```python
from build123d import *

# Parameters (mm, degrees)
BOSS_EXTRUDE1_DEPTH          = 44
SKETCH3_W                    = 50
SKETCH3_H                    = 50
BOSS_EXTRUDE2_DEPTH          = 11
SKETCH4_R                    = 21.25
SKETCH4_R_2                  = 12.25
CUT_EXTRUDE1_DEPTH           = 4
SKETCH5_3_R                  = 1.6
CUT_EXTRUDE3_DEPTH           = 20
SKETCH5_R                    = 2.5
CUT_EXTRUDE4_DEPTH           = 5
FILLET2_R                    = 15
SKETCH8_R                    = 3
CUT_EXTRUDE5_DEPTH           = 15
SCHIZZO2_W                   = 250
SCHIZZO2_H                   = 250
SCHIZZO2_W_2                 = 25.273765435
SCHIZZO2_H_2                 = 26.723899517
ESTRUSIONE_ESTRUSIONE1_DEPTH = 9
SCHIZZO5_W                   = 250
SCHIZZO5_H                   = 250
SCHIZZO5_W_2                 = 121.71
SCHIZZO5_H_2                 = 121.711825152
ESTRUSIONE_ESTRUSIONE2_DEPTH = 50


with BuildPart() as part:
    # Sketch1 → Boss-Extrude1 (new body)
    with BuildSketch(Plane.XY):
        Polygon((-22.5, 0), (22.5, 0), (18, 9), (-18, 9), align=None)
    extrude(amount=BOSS_EXTRUDE1_DEPTH)

    # Sketch3 → Boss-Extrude2 (add)
    with BuildSketch(Plane(origin=(0, 9, 0), x_dir=(1, 0, 0), z_dir=(0, 1, 0))):
        with Locations((0, -22)):
            Rectangle(SKETCH3_W, SKETCH3_H)
    extrude(amount=BOSS_EXTRUDE2_DEPTH)

    # Sketch4 → Cut-Extrude1 (cut)
    with BuildSketch(Plane(origin=(0, 20, 0), x_dir=(1, 0, 0), z_dir=(0, 1, 0))):
        with Locations((0, -22)):
            Circle(SKETCH4_R)
        with Locations((0, -22)):
            Circle(SKETCH4_R_2, mode=Mode.SUBTRACT)
    extrude(amount=-CUT_EXTRUDE1_DEPTH, mode=Mode.SUBTRACT)

    # Sketch5<3> → Cut-Extrude3 (cut)
    with BuildSketch(Plane(origin=(0, 20, 0), x_dir=(1, 0, 0), z_dir=(0, 1, 0))):
        with Locations((0, -15)):
            Circle(SKETCH5_3_R)
        with Locations((-7, -22)):
            Circle(SKETCH5_3_R)
        with Locations((7, -22)):
            Circle(SKETCH5_3_R)
        with Locations((0, -29)):
            Circle(SKETCH5_3_R)
    extrude(amount=-CUT_EXTRUDE3_DEPTH, mode=Mode.SUBTRACT)

    # Sketch5 → Cut-Extrude4 (cut)
    with BuildSketch(Plane(origin=(0, 20, 0), x_dir=(1, 0, 0), z_dir=(0, 1, 0))):
        with Locations((0, -22)):
            Circle(SKETCH5_R)
    extrude(amount=-CUT_EXTRUDE4_DEPTH, mode=Mode.SUBTRACT)

    # Fillet2
    fillet2_edges = [part.edges().sort_by_distance(p)[0] for p in [
        (25, 14.5, 47),
        (25, 14.5, -3),
        (-25, 14.5, -3),
        (-25, 14.5, 47),
    ]]
    fillet(fillet2_edges, radius=FILLET2_R)

    # Sketch8 → Cut-Extrude5 (cut)
    with BuildSketch(Plane(origin=(0, 0, 0), x_dir=(-1, 0, 0), z_dir=(0, -1, 0))):
        with Locations((0, -29)):
            Circle(SKETCH8_R)
        with Locations((-7, -22)):
            Circle(SKETCH8_R)
        with Locations((0, -15)):
            Circle(SKETCH8_R)
        with Locations((7, -22)):
            Circle(SKETCH8_R)
    extrude(amount=-CUT_EXTRUDE5_DEPTH, mode=Mode.SUBTRACT)

    # Schizzo2 → Estrusione-Estrusione1 (add)
    with BuildSketch(Plane.XZ):
        with Locations((0, 22)):
            Rectangle(SCHIZZO2_W, SCHIZZO2_H)
        with Locations((-0.310743018, 21.585675977)):
            Rectangle(SCHIZZO2_W_2, SCHIZZO2_H_2, mode=Mode.SUBTRACT)
    extrude(amount=-ESTRUSIONE_ESTRUSIONE1_DEPTH)

    # Schizzo5 → Estrusione-Estrusione2 (add)
    with BuildSketch(Plane.XZ):
        with Locations((0, 22)):
            Rectangle(SCHIZZO5_W, SCHIZZO5_H)
        with Locations((0, 22)):
            Rectangle(SCHIZZO5_W_2, SCHIZZO5_H_2, mode=Mode.SUBTRACT)
    extrude(amount=ESTRUSIONE_ESTRUSIONE2_DEPTH)


solid = part.part
```
Geometry check sheet. Reference: the model listing, model coordinates, mm. A direction names the side the tool comes from. Give positions to 0.01 mm unless a question says otherwise; leave off trailing zeros. Order: outer loops, then holes, each group sorted by start corner. A loop starts at its lowest first (then second) coordinate and runs counter-clockwise, first axis right, second up.
1. Access from +Z, -Z, +X, -X, +Y, -Y to the whole of each face (thin tool, end or side, straight path). Record for faces 4 (the face through (0, 14, 47)), 5 (the face through (-8.3, 15, 23.3)), 6 (the face through (0, 14, -3)).
2. Section check C-C, the plane x = 93.5. Enter the section's corners in (y, z).
3. Thickness scan on L1, parallel to Z at x = 0, y = 16.7; L2, parallel to X at y = 18.05, z = 22; L3, parallel to Z at x = 59, y = -35. Record the ranges inside material, lowest first.
4. Release check for a two-part mould opening along Z. For faces 1 (the face through (3, 20, 22)), 2 (the face through (4.23, 7.4, 23.15)), 3 (the face through (20.49, 14.58, 42.72)) record: pulls with the +Z half, pulls with the -Z half, needs draft (parallel to the pull), parting line crosses it, or undercut.
5. Section check B-B, the plane z = 115. Enter the section's corners in (x, y).
6. Gauge pin test, flat ends, axial feed: pin 1 Ø6.5 at (x, z) = (-1, 29.5) entering from -Y; pin 2 Ø5 at (x, z) = (-18.5, -56) entering from +Y; pin 3 Ø3.5 at (x, z) = (7, 22) entering from +Y; pin 4 Ø3.5 at (y, z) = (16.5, 24.5) entering from -X. Record the tip position at first contact, or that the pin passes through.
7. Section check A-A, the plane y = -11. Enter the section's corners in (x, z) (3 decimals).
Values follow:
1. face 4: +Z, +X, -X, +Y
1. face 5: -Y
1. face 6: -Z, +X, -X, +Y
2. outline: (-50, -103) - (9, -103) - (9, 147) - (-50, 147) - close
3. L1: z = -3 to 0.75, 9.75 to 13.4, 16.6 to 19.5, 24.5 to 27.4, 30.6 to 34.25, 43.25 to 47
3. L2: x = -25 to -21.25, -12.25 to -8.6, -5.4 to -2.5, 2.5 to 5.4, 8.6 to 12.25, 21.25 to 25
3. L3: z = -103 to -38.86, 82.86 to 147
4. face 1: needs draft
4. face 2: undercut
4. face 3: pulls with the +Z half
5. outline: (-125, -50) - (125, -50) - (125, 9) - (-125, 9) - close
6. pin 1: stops at y = 0
6. pin 2: stops at y = 9
6. pin 3: stops at y = 20
6. pin 4: stops at x = -25
7. outline: (-125, -103) - (125, -103) - (125, 147) - (-125, 147) - close; hole (-60.855, -38.856) - (60.855, -38.856) - (60.855, 82.856) - (-60.855, 82.856) - close
